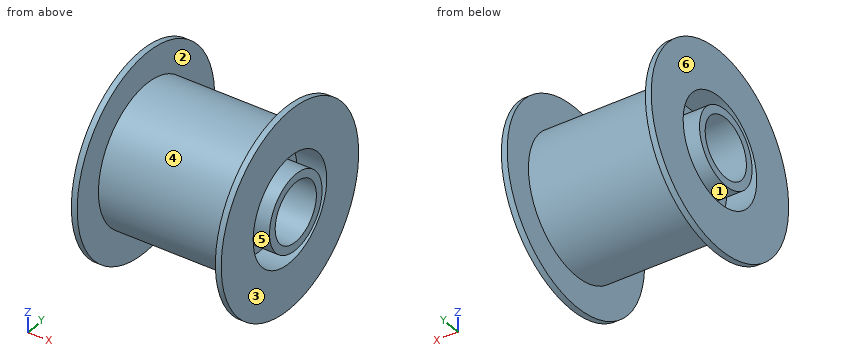
```python
from build123d import *


with BuildPart() as part:
    # Sketch1 → Revolve1 (revolve)
    with BuildSketch(Plane.XY, mode=Mode.PRIVATE) as revolve1_sk:
        Polygon((0, 6.5), (0, 5.1), (27.6, 5.1), (27.6, 6.5), (21.5, 6.5), (21.5, 9.1), (26.6, 9.1), (26.6, 17), (25.6, 17), (25.6, 11.75), (2, 11.75), (2, 17), (1, 17), (1, 9.1), (6.1, 9.1), (6.1, 6.5), align=None)
    revolve(revolve1_sk.sketch.rotate(Axis((0, 0, 0), (1, 0, 0)), 90), axis=Axis((0, 0, 0), (1, 0, 0)))


solid = part.part
```
Verification items for the finished model (mm, model axes). Face numbers are marked on the shaded views. A direction names the side the tool comes from. Round coordinates to 2 decimals unless told otherwise and drop trailing zeros. Order: outer loops, then holes, each group sorted by start corner. A loop starts at its lowest first (then second) coordinate and runs counter-clockwise, first axis right, second up.
1) Material ranges on line 1 (Y direction, x = 5.15, z = 0); line 2 (X direction, y = 14, z = -7.5); line 3 (Y direction, x = 9.75, z = 0), recorded low to high.
Geometry says:
line 1: y = -11.75 to -9.1, -6.5 to -5.1, 5.1 to 6.5, 9.1 to 11.75
line 2: x = 1 to 2, 25.6 to 26.6
line 3: y = -11.75 to -5.1, 5.1 to 11.75
2) Cross-section at D-D, the plane x = 12.25. Record the cut outline in (y, z), plus the area to 3 significant figures.
Geometry says:
outline: circle Ø23.5 at (0, 0); hole circle Ø10.2 at (0, 0)
area: 352 mm2
3) Cross-section at C-C, the plane x = 24.5. Record the cut outline in (y, z), plus the area to 3 significant figures.
Geometry says:
outline: circle Ø23.5 at (0, 0); circle Ø13 at (0, 0); hole circle Ø18.2 at (0, 0); hole circle Ø10.2 at (0, 0)
area: 225 mm2
4) Tool access check on the marked faces 1, 2 and 3. Record the directions out of +Z, -Z, +X, -X, +Y, -Y that give a thin tool (end or side, any length) a straight path to the whole face; none if there is none.
Geometry says:
face 1: -X
face 2: none
face 3: +X
5) Draft check along X on the marked faces 4, 5 and 6. Enter one of: +X half, -X half, draft (parallel to the pull), parting line (faces both ways), or undercut.
Geometry says:
face 4: undercut
face 5: draft
face 6: -X half
6) Depth check by flat-ended pin: pin 1 (3 mm diameter, centred on x = 9, z = -9, fed in from +Y) (3 decimals); pin 2 (1 mm diameter, centred on x = 5, z = -1.5, fed in from +Y); pin 3 (2 mm diameter, centred on x = 21, y = -11, fed in from -Z); pin 4 (1.5 mm diameter, centred on y = -3, z = 1.5, fed in from -X). Enter the tip coordinate at first touch or a pass-through.
Geometry says:
pin 1: stops at y = 9.045
pin 2: stops at y = 11.71
pin 3: stops at z = -6.17
pin 4: passes through
